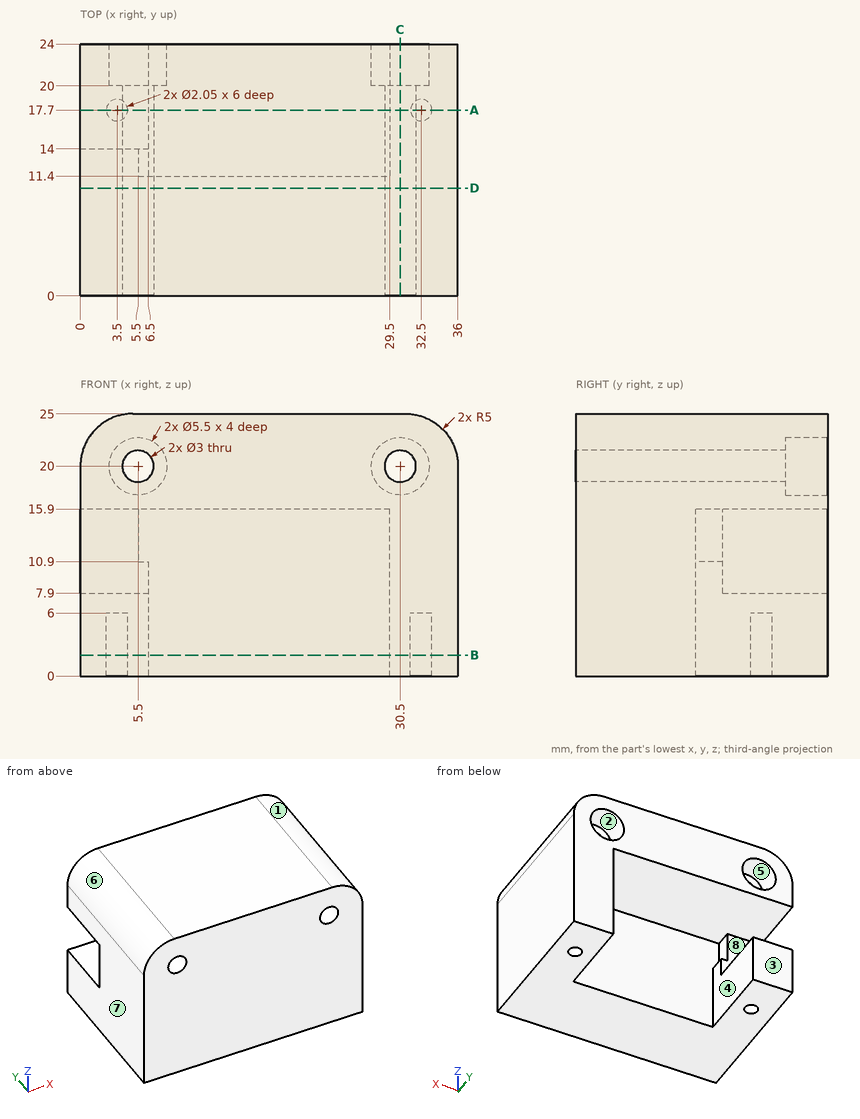
Verification items for this drawing (mm, ordinates from the low corner). A direction names the side the tool comes from. Round coordinates to 2 decimals unless told otherwise and drop trailing zeros. Write each loop counter-clockwise with the first axis right and the second up, starting at its lowest first coordinate (ties: lowest second). Pieces come first, ordered by that corner, then holes. Notation, with made-up numbers: M 79.5,75.25 L 123.5,75.25 A23 cw 123.5,101.25 Z; hole C 24,16.25 d4. An arc over 180 degrees is marked long. Write item = value, one per line. Start each with the question number.
1. Scan lines: line 1 (X direction, y = 21, z = 20); line 2 (Z direction, x = 5.5, y = 21); line 3 (Z direction, x = 5.5, y = 9.25). Record each from-to range of solid material in increasing order. Write a range as [from, to].
2. Tool access check on the marked faces 4, 5, 6, 7 and 8. Record the directions out of +Z, -Z, +X, -X, +Y, -Y that give a thin tool (end or side, any length) a straight path to the whole face; none if there is none.
3. Release check for a two-part mould opening along Z. For the marked faces 1, 2 and 3 record: pulls with the +Z half, pulls with the -Z half, needs draft (parallel to the pull), parting line crosses it, or undercut.
4. Section check A-A, the plane y = 17.7. Record the cut outline in (x, z) (3 decimals).
5. Section check C-C, the plane x = 30.5. Record the cut outline in (y, z).
6. Section check D-D, the plane y = 10.25. Record the cut outline in (x, z), then the cut area to 3 significant figures.
7. Section check B-B, the plane z = 2. Record the cut outline in (x, y) (3 decimals), then the cut area to 3 significant figures.
8. Gauge pin test, flat ends, axial feed: pin 1 (2.5 mm diameter, centred on x = 30.5, z = 20, fed in from +Y); pin 2 (4 mm diameter, centred on x = 10.5, y = 17, fed in from -Z); pin 3 (2.5 mm diameter, centred on x = 6, z = 20, fed in from +Y); pin 4 (5 mm diameter, centred on x = 4.5, z = 11, fed in from +Y). Record the tip position at first contact, or that the pin passes through.
Results found:
q1.line_1 = [0, 2.75], [8.25, 27.75], [33.25, 36]
q1.line_2 = [0, 7.9], [15.9, 17.25], [22.75, 25]
q1.line_3 = [0, 18.5], [21.5, 25]
q2.face_4 = -Z, +Y
q2.face_5 = +Y
q2.face_6 = +Z, -X, +Y, -Y
q2.face_7 = +Z, -Z, -X, +Y, -Y
q2.face_8 = -X, +Y
q3.face_1 = pulls with the +Z half
q3.face_2 = undercut
q3.face_3 = needs draft
q4.outline = M 0,0 L 2.475,0 L 2.475,6 L 4.525,6 L 4.525,0 L 6.5,0 L 6.5,7.9 L 0,7.9 Z; M 0,15.9 L 29.5,15.9 L 29.5,0 L 31.475,0 L 31.475,6 L 33.525,6 L 33.525,0 L 36,0 L 36,20 A5 ccw 31,25 L 5,25 A5 ccw 0,20 Z; hole C 5.5,20 d3; hole C 30.5,20 d3
q5.outline = M 0,0 L 24,0 L 24,17.25 L 20,17.25 L 20,18.5 L 0,18.5 Z; M 0,21.5 L 20,21.5 L 20,22.75 L 24,22.75 L 24,25 L 0,25 Z
q6.outline = M 0,0 L 36,0 L 36,20 A5 ccw 31,25 L 5,25 A5 ccw 0,20 Z; hole C 5.5,20 d3; hole C 30.5,20 d3
q6.area = 875 mm^2
q7.outline = M 0,0 L 36,0 L 36,24 L 29.5,24 L 29.5,11.4 L 6.5,11.4 L 6.5,24 L 0,24 Z; hole C 3.5,17.7 d2.05; hole C 32.5,17.7 d2.05
q7.area = 568 mm^2
q8.pin_1 = through
q8.pin_2 = 15.9
q8.pin_3 = 20
q8.pin_4 = 14
